The model under review builds one solid part; all positions refer to its coordinate system, in mm. A direction names the side the tool comes from. Give positions to 0.01 mm unless a question says otherwise; leave off trailing zeros. Order: outer loops, then holes, each group sorted by start corner. A loop starts at its lowest first (then second) coordinate and runs counter-clockwise, first axis right, second up. Notation, with made-up numbers: (47.5, -1.5) - (53.5, -1.5) arc R26 ccw to (53.5, 16.5) - close; hole circle Ø1 at (66.25, -27). An arc over 180 degrees is marked (long way). Answer as CSV lines item,"result". Start each with the question number.
Autodesk Inventor part; units mm, degrees
ref_plane "YZ Plane" through (0, 0, 0) normal (1, 0, 0) x (0, 1, 0)
ref_plane "XZ Plane" through (0, 0, 0) normal (0, 1, 0) x (-1, 0, 0)
ref_plane "XY Plane" through (0, 0, 0) normal (0, 0, 1) x (1, 0, 0)
sketch "Sketch1" plane through (0, 0, 0) normal (0, 0, 1) x (1, 0, 0)
  line L0 (-12.1708, 16.0073) -> (13.2292, 16.0073)
  line L1 (13.2292, 16.0073) -> (13.2292, -34.7927)
  line L2 (13.2292, -34.7927) -> (-12.1708, -34.7927)
  line L3 (-12.1708, -34.7927) -> (-12.1708, 16.0073)
  line L4 (11.9592, 14.7373) -> (-10.9008, 14.7373)
  line L5 (-10.9008, 14.7373) -> (-10.9008, -33.5227)
  line L6 (-10.9008, -33.5227) -> (11.9592, -33.5227)
  line L7 (11.9592, -33.5227) -> (11.9592, 14.7373)
  point P0 (0, 0)
  dimension "d0" = 25.4
  dimension "d1" = 50.8
  dimension "d2" = 1.27
extrude "Extrusion1" add sketch "Sketch1" along normal blind 114.935
sketch "Sketch2" plane through (-12.1708, 16.0073, 0) normal (0, 1, 0) x (1, 0, 0)
  circle A0 centre (12.7, -12.7) radius 1.7272
  line L0 (25.4, 0) -> (0, 0)
  line L1 (0, 0) -> (0, -114.935)
  point P0 (12.1708, 0)
  dimension "d5" = 3.4544
  dimension "d6" = 12.7
  dimension "d7" = 12.7
extrude "Extrusion2" cut sketch "Sketch2" against normal through all
pattern_linear "Rectangular Pattern1" count 11 spacing 25.4 along (0, 0, 1) of "Extrusion2"
sketch "Sketch3" plane through (13.2292, -34.7927, 0) normal (1, 0, 0) x (0, 0, -1)
  circle A0 centre (-80.645, 25.4) radius 14.2875
  line L0 (0, 0) -> (0, 50.8)
  line L1 (-114.935, 0) -> (-114.935, 50.8)
  point P0 (0, 34.7927)
  dimension "d15" = 28.575
  dimension "d20" = 80.645
extrude "Extrusion3" cut sketch "Sketch3" against normal through all
equation "\"d3\" = d13"
equation "\"d10\" = d14"
equation "\"d13\" = 114.935"
equation "\"d14\" = d13"
properties part number "VerseFrame 5in STOCK"
Item 1: For line 1 along X through (y, z) = (-33.95, 114.3); line 2 along Y through (x, z) = (-3.5, 5); line 3 along X through (y, z) = (9, 92), list the stretches that pass through material, from the lowest coordinate up.
Item 2: Take a section at C-C on y = -30.5. Write out the cut boundary in (x, z) (3 decimals), and give its area (3 significant figures).
Item 3: Take a section at A-A on z = 38.1. Write out the cut boundary in (x, y).
Item 4: Machinability: for faces 4 (the face through (0, -33.523, 57)), 5 (the face through (0.3, 15.38, 61.79)), which of the approach directions +Z, -Z, +X, -X, +Y, -Y give a long, thin tool a straight path to every point of the face, cutting with its end or side? Answer none if there is none.
Item 5: Take a section at D-D on z = 88.9. Write out the cut boundary in (x, y), and give its area (3 significant figures).
Item 6: Clearance check with a flat-ended pin moving along its axis: pin 1 (23 mm diameter, centred on y = -9.39, z = 80.64, fed in from +X). State where the tip first meets the part, or that it passes through.
Item 7: Mouldability with a two-part tool opening along X and no side actions: class faces 1 (the face through (12.6, -8.76, 94.92)), 2 (the face through (13.229, -9, 57)), 3 (the face through (0.3, 15.38, 87.19)) as released by +X, released by -X, zero draft, split by the parting line, or undercut.
Item 8: Take a section at B-B on x = 9.5. Write out the cut boundary in (y, z) (3 decimals).
Data:
1,line 1,"x = -12.17 to -1.2, 2.26 to 13.23"
1,line 2,"y = -34.79 to -33.52, 14.74 to 16.01"
1,line 3,"x = -12.17 to -10.9, 11.96 to 13.23"
2,outline,"(-12.171, 0) - (-10.901, 0) - (-10.901, 114.935) - (-12.171, 114.935) - close; (11.959, 0) - (13.229, 0) - (13.229, 114.935) - (11.959, 114.935) - close"
2,area,"292 mm^2"
3,outline,"(-12.17, -34.79) - (-1.2, -34.79) - (-1.2, -33.52) - (-10.9, -33.52) - (-10.9, 14.74) - (-1.2, 14.74) - (-1.2, 16.01) - (-12.17, 16.01) - close; (2.26, -34.79) - (13.23, -34.79) - (13.23, 16.01) - (2.26, 16.01) - (2.26, 14.74) - (11.96, 14.74) - (11.96, -33.52) - (2.26, -33.52) - close"
4,face 4,"+Z, -Z"
4,face 5,"+Y, -Y"
5,outline,"(-12.17, -34.79) - (-1.2, -34.79) - (-1.2, -33.52) - (-10.9, -33.52) - (-10.9, -21.05) - (-12.17, -21.05) - close; (-12.17, 2.27) - (-10.9, 2.27) - (-10.9, 14.74) - (-1.2, 14.74) - (-1.2, 16.01) - (-12.17, 16.01) - close; (2.26, -34.79) - (13.23, -34.79) - (13.23, -21.05) - (11.96, -21.05) - (11.96, -33.52) - (2.26, -33.52) - close; (2.26, 14.74) - (11.96, 14.74) - (11.96, 2.27) - (13.23, 2.27) - (13.23, 16.01) - (2.26, 16.01) - close"
5,area,"119 mm^2"
6,pin 1,"passes through"
7,face 1,"zero draft"
7,face 2,"released by +X"
7,face 3,"undercut"
8,outline,"(-34.793, 0) - (-33.523, 0) - (-33.523, 114.935) - (-34.793, 114.935) - close; (14.737, 0) - (16.007, 0) - (16.007, 114.935) - (14.737, 114.935) - close"
